from build123d import *

# Parameters (mm, degrees)
SKETCH1_W           = 5.4864
SKETCH1_H           = 50.8
CUT_EXTRUDE1_DEPTH  = 14.732
CUT_EXTRUDE2_DEPTH  = 14.732
SKETCH4_R           = 3.175
BOSS_EXTRUDE1_DEPTH = 7.9248
SKETCH5_R           = 2.4511
BOSS_EXTRUDE2_DEPTH = 6.858


with BuildPart() as part:
    # Sketch1 → Revolve1 (revolve)
    with BuildSketch(Plane.XY, mode=Mode.PRIVATE) as revolve1_sk:
        with Locations((628.657823135, 122.745244002)):
            Rectangle(SKETCH1_W, SKETCH1_H)
    revolve(revolve1_sk.sketch.rotate(Axis((625.914623135, 148.145244002, 0), (0, -1, 0)), 270), axis=Axis((625.914623135, 148.145244002, 0), (0, -1, 0)))

    # Sketch2 → Cut-Extrude1 (cut)
    with BuildSketch(Plane(origin=(0, 148.145244002, 0), x_dir=(-1, 0, 0), z_dir=(0, 1, 0))):
        with BuildLine():
            Line((-628.028719536, 5.062724698), (-620.473126733, 0.700501159))
            ThreePointArc((-620.473126733, 0.700501159), (-623.171423135, 4.751361775), (-628.028719536, 5.062724698))
        make_face()
    extrude(amount=-CUT_EXTRUDE1_DEPTH, mode=Mode.SUBTRACT)

    # Sketch3 → Cut-Extrude2 (cut)
    with BuildSketch(Plane(origin=(0, 148.145244002, 0), x_dir=(-1, 0, 0), z_dir=(0, 1, 0))):
        with BuildLine():
            Line((-623.800526733, -5.062724698), (-631.356119536, -0.700501159))
            ThreePointArc((-631.356119536, -0.700501159), (-628.657823135, -4.751361775), (-623.800526733, -5.062724698))
        make_face()
    extrude(amount=-CUT_EXTRUDE2_DEPTH, mode=Mode.SUBTRACT)

    # Sketch4 → Boss-Extrude1 (add)
    with BuildSketch(Plane(origin=(0, 148.145244002, 0), x_dir=(-1, 0, 0), z_dir=(0, 1, 0))):
        with Locations(Location((-625.914623135, 0, 0), (0, 0, 90))):
            Circle(SKETCH4_R)
    extrude(amount=BOSS_EXTRUDE1_DEPTH)

    # Sketch5 → Boss-Extrude2 (add)
    with BuildSketch(Plane(origin=(0, 156.070044002, 0), x_dir=(-1, 0, 0), z_dir=(0, 1, 0))):
        with Locations(Location((-625.914623135, 0, 0), (0, 0, 270))):
            Circle(SKETCH5_R)
    extrude(amount=BOSS_EXTRUDE2_DEPTH)


solid = part.part
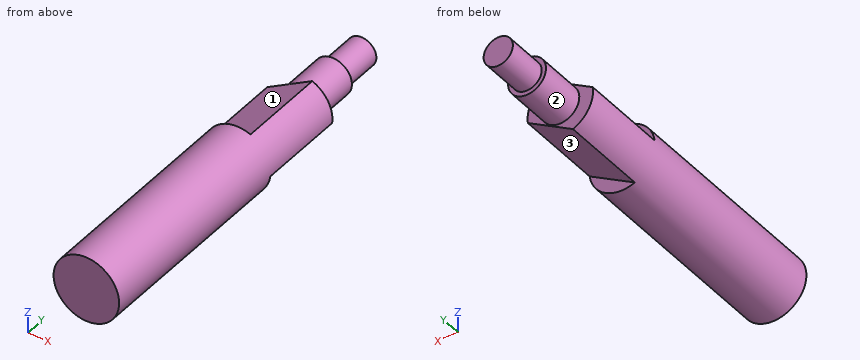
Source: CAD feature listing. Evaluate the final solid. Frame: model axes, mm. Face numbers are marked on the shaded views. A direction names the side the tool comes from. Coordinates: 2 decimals unless noted, no trailing zeros. Loops run counter-clockwise (first coordinate to the right, second up) from the corner with the lowest first, then second, coordinate; pieces in that order, holes last. Notation, with made-up numbers: (32, 65) - (45, 65) arc R22 ccw to (45, 98) - close; hole circle Ø7 at (-9.5, 76.25). An arc over 180 degrees is marked (long way). One line per question, with ' | ' between items.
1) Section D-D, the plane x = 627.25. Return loops of the section in (y, z), then the cut area to 3 significant figures.
Report:
outline: (97.35, -5.32) - (133.41, -5.32) - (133.41, -3.07) - (148.15, -3.07) - (148.15, -2.88) - (156.07, -2.88) - (156.07, -2.06) - (162.93, -2.06) - (162.93, 2.06) - (156.07, 2.06) - (156.07, 2.88) - (148.15, 2.88) - (148.15, 4.61) - (133.41, 4.61) - (133.41, 5.32) - (97.35, 5.32) - close | area: 571 mm²
2) Set-up query: the marked faces 1, 2 and 3. Return all of +Z, -Z, +X, -X, +Y, -Y with unobstructed straight access to the full face (end or side cutting, diameter ignored); none if empty.
Report:
face 1: +Z, -X, +Y | face 2: +Y | face 3: -Z, +X, +Y
3) Section C-C, the plane x = 624.5. Return loops of the section in (y, z).
Report:
outline: (97.35, -5.3) - (133.41, -5.3) - (133.41, -4.66) - (148.15, -4.66) - (148.15, -2.84) - (156.07, -2.84) - (156.07, -2) - (162.93, -2) - (162.93, 2) - (156.07, 2) - (156.07, 2.84) - (148.15, 2.84) - (148.15, 3.03) - (133.41, 3.03) - (133.41, 5.3) - (97.35, 5.3) - close
4) Line query: line 1 along Y through (x, z) = (631, 0.5); line 2 along Y through (x, z) = (625.75, -4.25); line 3 along X through (y, z) = (149, -0.25). Output: solid intervals per line, ascending.
Report:
line 1: y = 97.35 to 148.15 | line 2: y = 97.35 to 133.41 | line 3: x = 622.75 to 629.08
5) First-contact query: P1, Ø1, axis at y = 117, z = -1, coming from the +X side; P2, Ø1.5, axis at x = 627.5, y = 152, coming from the -Z side; P3, Ø1.4, axis at x = 629, z = -3.5, coming from the +Y side. Flat tips, straight axial feed; report the tip coordinate or a pass-through.
Report:
P1: stops at x = 631.38 | P2: stops at z = -3.06 | P3: stops at y = 133.41
6) Section B-B, the plane y = 146.5. Return loops of the section in (x, z), then the cut area to 3 significant figures.
Report:
outline: (620.47, 0.7) arc R5.49 ccw to (623.8, -5.06) - (631.36, -0.7) arc R5.49 ccw to (628.03, 5.06) - close | area: 68.3 mm²
7) Section A-A, the plane z = 0. Return loops of the section in (x, y), then the cut area to 3 significant figures.
Report:
outline: (620.43, 97.35) - (631.4, 97.35) - (631.4, 148.15) - (629.09, 148.15) - (629.09, 156.07) - (628.37, 156.07) - (628.37, 162.93) - (623.46, 162.93) - (623.46, 156.07) - (622.74, 156.07) - (622.74, 148.15) - (620.43, 148.15) - close | area: 641 mm²
